Model file for the job. Use its own axes, mm. Give positions to 0.01 mm unless a question says otherwise; leave off trailing zeros. Loops run counter-clockwise (first coordinate to the right, second up) from the corner with the lowest first, then second, coordinate; pieces in that order, holes last. Notation, with made-up numbers: M 45.5,-31.75 L 101.5,-31.75 A12 ccw 101.5,-13.75 Z; hole C -36,4 d9. An arc over 180 degrees is marked long. Answer in a Markdown table with one row per item.
```python
from build123d import *

# Parameters (mm, degrees)
SKETCH1_R           = 165.1
BOSS_EXTRUDE1_DEPTH = 203.2
REVOLVE1_ANGLE      = 180
SHELL1_T            = -2.54


with BuildPart() as part:
    # Sketch1 → Boss-Extrude1 (new body)
    with BuildSketch(Plane(origin=(0, 0, 0), x_dir=(1, 0, 0), z_dir=(0, 1, 0))):
        with Locations(Location((0, 0, 0), (0, 0, 270))):
            Circle(SKETCH1_R)
    extrude(amount=BOSS_EXTRUDE1_DEPTH)

    # Sketch2 → Revolve1 (revolve)
    with BuildSketch(Plane(origin=(0, 203.2, 0), x_dir=(1, 0, 0), z_dir=(0, 1, 0))):
        with BuildLine():
            Line((0, 165.1), (0, -165.1))
            ThreePointArc((0, -165.1), (165.1, 0), (0, 165.1))
        make_face()
    revolve(axis=Axis((0, 203.2, -165.1), (0, 0, 1)), revolution_arc=REVOLVE1_ANGLE)

    # Shell1
    shell1_openings = [part.faces().sort_by_distance(p)[0] for p in [
        (0, 0, 0),
    ]]
    offset(amount=SHELL1_T, openings=shell1_openings, kind=Kind.INTERSECTION)


solid = part.part
```
Q1. Saw through at A-A (z = 0). Give the cut face in (x, y).
Reported:
| item | result |
|---|---|
| outline | M -165.1,0 L -162.56,0 L -162.56,203.2 A162.56 cw 162.56,203.2 L 162.56,0 L 165.1,0 L 165.1,203.2 A165.1 ccw -165.1,203.2 Z |
Q2. Drop flat-ended pins along their axis: pin 1 (1.5 mm diameter, centred on x = 6, y = 248.5, fed in from -Z); pin 2 (1 mm diameter, centred on x = 27.5, z = -32.5, fed in from +Y); pin 3 (1.5 mm diameter, centred on x = 85.5, y = 199.5, fed in from +Z). Give the stop position or say it passes through.
Reported:
| item | result |
|---|---|
| pin 1 | z = -158.86 |
| pin 2 | y = 362.85 |
| pin 3 | z = 141.69 |
Q3. Mould opens along Z. For faces 1 (the face through (161.177, 100.178, -21.162)), 2 (the face through (163.695, 100.178, -21.493)), 3 (the face through (-109, 0, 122)) say: released by +Z, released by -Z, zero draft, split by the parting line, or undercut.
Reported:
| item | result |
|---|---|
| face 1 | undercut |
| face 2 | split by the parting line |
| face 3 | zero draft |
Q4. Probe probe 1 along X at (y, z) = (150.5, 0); probe 2 along Z at (x, y) = (-90, 304.5). List the from-to ranges inside material, lowest first.
Reported:
| item | result |
|---|---|
| probe 1 | -165.1 to -162.56, 162.56 to 165.1 |
| probe 2 | -94.32 to -89.8, 89.8 to 94.32 |
Q5. Saw through at B-B (x = 0). Give the cut face in (y, z), and give its area (3 significant figures).
Reported:
| item | result |
|---|---|
| outline | M 0,-165.1 L 203.2,-165.1 A165.1 ccw 203.2,165.1 L 0,165.1 L 0,162.56 L 203.2,162.56 A162.56 cw 203.2,-162.56 L 0,-162.56 Z |
| area | 2,340 mm² |
Q6. Saw through at C-C (y = 189). Give the cut face in (x, z), and give its area (3 significant figures).
Reported:
| item | result |
|---|---|
| outline | C 0,0 d330.2; hole C 0,0 d325.12 |
| area | 2,610 mm² |
